Source: CAD feature listing. Evaluate the final solid. Frame: model axes, mm. A direction names the side the tool comes from. Round coordinates to 2 decimals unless told otherwise and drop trailing zeros. Loops run counter-clockwise (first coordinate to the right, second up) from the corner with the lowest first, then second, coordinate; pieces in that order, holes last.
Item 1: Section query B-B on y = 6. Return loops of the section in (x, z), then the cut area to 3 significant figures.
Item 2: Section query D-D on y = 36. Return loops of the section in (x, z), then the cut area to 3 significant figures.
Item 3: Section query A-A on x = 0. Return loops of the section in (y, z), then the cut area to 3 significant figures.
Item 4: Pull-direction query (X, two-part tool) for faces 1 (the cylindrical face through (-18.23, 19.85, 3.04)), 2 (the cylindrical face through (-44.96, 1.94, 2.96)), 3 (the flat face through (-11, 11, 0)); classes: released by +X, released by -X, zero draft, split by the parting line, or undercut.
Item 5: Access query for faces 4 (the cylindrical face through (-14.288, 0.586, 2.958)), 5 (the flat face through (29, -3, 3)). Directions: +Z, -Z, +X, -X, +Y, -Y. A direction counts if a zero-diameter tool reaches every point of the face in a straight line with its end or side. Return the directions, or none.
Item 6: Section query C-C on z = 1.75. Return loops of the section in (x, y), then the cut area to 3 significant figures.
Item 7: First-contact query: P1, Ø3, axis at x = 26.5, z = 4, coming from the +Y side; P2, Ø2, axis at y = -27, z = 1, coming from the +X side; P3, Ø2, axis at x = 2, z = 3.5, coming from the -Y side. Flat tips, straight axial feed; report the tip coordinate or a pass-through.
Item 8: Ray query, L1, parallel to X at y = -22, z = 1.8; L2, parallel to Y at x = 21.5, z = 2; L3, parallel to Y at x = 23, z = 5.3. Return the intervals inside material, ascending.
```python
from build123d import *

# Parameters (mm, degrees)
SKETCH_R        = 45
SKETCH_R_2      = 14.3
PAD_DEPTH       = 6
SKETCH001_R     = 3
POCKET_DEPTH    = 10
SKETCH002_W     = 50
SKETCH002_H     = 6
POCKET001_DEPTH = 10


with BuildPart() as part:
    # Sketch → Pad (new body)
    with BuildSketch(Plane.XY):
        Circle(SKETCH_R)
        Circle(SKETCH_R_2, mode=Mode.SUBTRACT)
    extrude(amount=PAD_DEPTH)

    # Sketch001 → Pocket (cut)
    with BuildSketch(Plane.XY.offset(6)):
        with Locations((-21.001071, 21.001071)):
            Circle(SKETCH001_R)
        with Locations((21.001071, 21.001071)):
            Circle(SKETCH001_R)
        with Locations((-21.001071, -21.001071)):
            Circle(SKETCH001_R)
        with Locations((21.001071, -21.001071)):
            Circle(SKETCH001_R)
    extrude(amount=-POCKET_DEPTH, mode=Mode.SUBTRACT)

    # Sketch002 → Pocket001 (cut)
    with BuildSketch(Plane.XY.offset(6)):
        with Locations((25, 0)):
            Rectangle(SKETCH002_W, SKETCH002_H)
    extrude(amount=-POCKET001_DEPTH, mode=Mode.SUBTRACT)


solid = part.part
```
Data:
1. outline: (-44.6, 0) - (-12.98, 0) - (-12.98, 6) - (-44.6, 6) - close; (12.98, 0) - (44.6, 0) - (44.6, 6) - (12.98, 6) - close
1. area: 379 mm2
2. outline: (-27, 0) - (27, 0) - (27, 6) - (-27, 6) - close
2. area: 324 mm2
3. outline: (-45, 0) - (-14.3, 0) - (-14.3, 6) - (-45, 6) - close; (14.3, 0) - (45, 0) - (45, 6) - (14.3, 6) - close
3. area: 368 mm2
4. face 1: undercut
4. face 2: split by the parting line
4. face 3: zero draft
5. face 4: +Z, -Z
5. face 5: +Z, -Z, +X
6. outline: (13.98, -3) arc R14.3 cw (long way) to (13.98, 3) - (44.9, 3) arc R45 ccw (long way) to (44.9, -3) - close; hole circle Ø6 at (-21, -21); hole circle Ø6 at (-21, 21); hole circle Ø6 at (21, -21); hole circle Ø6 at (21, 21)
6. area: 5,420 mm2
7. P1: stops at y = 37.42
7. P2: stops at x = 36.73
7. P3: stops at y = -44.99
8. L1: x = -39.26 to -23.83, -18.17 to 18.17, 23.83 to 39.26
8. L2: y = -39.53 to -23.96, -18.04 to -3, 3 to 18.04, 23.96 to 39.53
8. L3: y = -38.68 to -23.24, -18.76 to -3, 3 to 18.76, 23.24 to 38.68
